CAD build for the part. Positions are in the model's coordinates, mm. Give positions to 0.01 mm unless a question says otherwise; leave off trailing zeros. Order: outer loops, then holes, each group sorted by start corner. A loop starts at its lowest first (then second) coordinate and runs counter-clockwise, first axis right, second up. Notation, with made-up numbers: M 87,15.5 L 103,15.5 A4 ccw 103,20.5 Z; hole C 46,20.25 d4. An arc over 180 degrees is marked long. Put each result on its own line as item: value. Start each with the question number.
1) Cut at C-C (x = 31.25). Write the cut outline in (y, z).
2) Cut at A-A (y = 21). Write the cut outline in (x, z).
3) Drill centre lines: line 1 (Y direction, x = 29.35, z = -19.5); line 2 (Z direction, x = 31.1, y = 21.5); line 3 (Y direction, x = 27.7, z = -19). Where is each one in solid material? Low to high. Write a range as [from, to].
4) Two-plate mould, pull along Z, no slides. Class faces 1 (the face through (29.472, 24.966, -18.979)), 2 (the face through (27.5, 18, -19)), 3 (the face through (29, 23, -18)): released by +Z, released by -Z, zero draft, split by the parting line, or undercut.
5) Cut at D-D (z = -22.5). Write the cut outline in (x, y), and give its area (3 significant figures).
6) Pin check, flat tips, straight feed: pin 1 (1 mm diameter, centred on x = 29.5, y = 24, fed in from +Z); pin 2 (2 mm diameter, centred on x = 28.5, z = -17.5, fed in from +Y); pin 3 (1 mm diameter, centred on x = 28.5, z = -22, fed in from +Y). Stop position of each tip, or through.
7) Cut at B-B (z = -19.5). Write the cut outline in (x, y), and give its area (3 significant figures).
```python
from build123d import *

# Parameters (mm, degrees)
CYLINDER014_R     = 2.5
CYLINDER014_DEPTH = 10
CYLINDER015_R     = 4
CYLINDER015_DEPTH = 4


with BuildPart() as cylinder002:
    # Cylinder014 → Cylinder014 (new body)
    with BuildSketch(Plane(origin=(23.5, -39, -22), x_dir=(0, 0, -1), z_dir=(1, 0, 0))):
        Circle(CYLINDER014_R)
    extrude(amount=CYLINDER014_DEPTH)


with BuildPart() as obj1:
    # Cylinder015 → Cylinder015 (new body)
    with BuildSketch(Plane(origin=(26.5, -39, -22), x_dir=(0, 0, -1), z_dir=(1, 0, 0))):
        Circle(CYLINDER015_R)
    extrude(amount=CYLINDER015_DEPTH)

    # Cut008: cut Cylinder002
    add(cylinder002.part, mode=Mode.SUBTRACT)


with BuildPart() as obj1_1:
    # Cut008 placement: moved
    add(obj1.part.moved(Location((1, 60, 2.5))))


solid = obj1_1.part
```
Solution:
1. outline: C 21,-19.5 d8; hole C 21,-19.5 d5
2. outline: M 27.5,-23.5 L 31.5,-23.5 L 31.5,-22 L 27.5,-22 Z; M 27.5,-17 L 31.5,-17 L 31.5,-15.5 L 27.5,-15.5 Z
3. line 1: [17, 18.5], [23.5, 25]
3. line 2: [-23.47, -21.95], [-17.05, -15.53]
3. line 3: [17.03, 18.55], [23.45, 24.97]
4. face 1: split by the parting line
4. face 2: zero draft
4. face 3: undercut
5. outline: M 27.5,18.35 L 31.5,18.35 L 31.5,23.65 L 27.5,23.65 Z
5. area: 21.2 mm²
6. pin 1: z = -16.38
6. pin 2: y = 24.87
6. pin 3: y = 24.46
7. outline: M 27.5,17 L 31.5,17 L 31.5,18.5 L 27.5,18.5 Z; M 27.5,23.5 L 31.5,23.5 L 31.5,25 L 27.5,25 Z
7. area: 12.0 mm²
